from build123d import *

# Parameters (mm, degrees)
F0_R     = 17.283329
F0_R_2   = 8.664102
F1_DEPTH = 30


with BuildPart() as f1:
    # F0 (on Front) → F1 (new body)
    with BuildSketch(Plane.XZ):
        with BuildLine():
            ThreePointArc((-53.428299, -27.878553), (-36.62345, -18.213297), (-29.982977, 0))
            ThreePointArc((-29.982977, 0), (-36.62345, 18.213297), (-53.428299, 27.878553))
            ThreePointArc((-53.428299, 27.878553), (-86.578354, 0), (-53.428299, -27.878553))
        make_face()
        with Locations((-58.280665, 0)):
            Circle(F0_R, mode=Mode.SUBTRACT)
        with BuildLine():
            ThreePointArc((-53.428299, 27.878553), (-36.62345, 18.213297), (-29.982977, 0))
            ThreePointArc((-29.982977, 0), (-36.62345, -18.213297), (-53.428299, -27.878553))
            Line((-53.428299, -27.878553), (59.125109, -15.380887))
            ThreePointArc((59.125109, -15.380887), (41.996, -1.293634), (56.538776, 15.450461))
            Line((56.538776, 15.450461), (-53.428299, 27.878553))
        make_face()
        with BuildLine():
            ThreePointArc((72.892666, 0), (68.044897, 11.249072), (56.538776, 15.450461))
            ThreePointArc((56.538776, 15.450461), (41.996, -1.293634), (59.125109, -15.380887))
            ThreePointArc((59.125109, -15.380887), (68.948042, -10.321305), (72.892666, 0))
        make_face()
        with Locations((57.417251, 0)):
            Circle(F0_R_2, mode=Mode.SUBTRACT)
    extrude(amount=F1_DEPTH)


solid = f1.part
Work out the finished part from the listing and answer in its coordinate system (mm). Give positions to 0.01 mm unless a question says otherwise; leave off trailing zeros. Order: outer loops, then holes, each group sorted by start corner. A loop starts at its lowest first (then second) coordinate and runs counter-clockwise, first axis right, second up. Notation, with made-up numbers: (24, 82) -> (77, 82) arc R13 ccw to (77, 106) -> close; hole circle Ø2 at (15.5, -26). An arc over 180 degrees is marked (long way). One line per item, written item: value.
Item 1: Find section D-D, the plane x = -7.5. Give the vertices of the cut face in (y, z).
Answer sheet:
outline: (-30, -22.78) -> (0, -22.78) -> (0, 22.69) -> (-30, 22.69) -> close
Item 2: Determine the mould class of faces 1 (the flat face through (-8, -30, 0)), 2 (the cylindrical face through (55.54, -14.79, -8.46)), 3 (the flat face through (2.061, -14.79, -21.717)) for opening direction X: released by +X, released by -X, zero draft, split by the parting line, or undercut.
Answer sheet:
face 1: zero draft
face 2: undercut
face 3: released by +X
Item 3: Straight lines are drawn through the part: probe 1 along X at (y, z) = (-17, -3); probe 2 along X at (y, z) = (-27.5, -9); probe 3 along X at (y, z) = (-3.5, -6). For each, find the intervals that lie inside material, in ascending order.
Answer sheet:
probe 1: -86.42 to -75.3, -41.26 to 49.29, 65.55 to 72.6
probe 2: -85.11 to -73.04, -43.53 to 70.01
probe 3: -85.93 to -74.49, -42.07 to 51.17, 63.67 to 71.68
Item 4: Flat-ended cylindrical pins translate along their axes: P1, Ø1.5, axis at y = -4.5, z = 15, coming from the -X side; P2, Ø3, axis at x = 26, y = -6, coming from the -Z side; P3, Ø8, axis at x = -17.5, y = -13, coming from the -Z side. Find the tip coordinate at first contact, or state that the pin passes through.
Answer sheet:
P1: x = -82.73
P2: z = -19.23
P3: z = -24.33
Item 5: Find section B-B, the plane x = -48.5. Give the vertices of the cut face in (y, z), plus the area to 3 significant figures.
Answer sheet:
outline: (-30, -27.33) -> (0, -27.33) -> (0, -14.25) -> (-30, -14.25) -> close; (-30, 14.25) -> (0, 14.25) -> (0, 27.32) -> (-30, 27.32) -> close
area: 785 mm²
Item 6: Find section A-A, the plane y = -24.25. Give the vertices of the cut face in (x, z), plus the area to 3 significant figures.
Answer sheet:
outline: (-53.43, -27.88) -> (59.13, -15.38) arc R15.48 ccw to (72.89, 0) arc R15.48 ccw to (56.54, 15.45) -> (-53.43, 27.88) arc R28.3 ccw (long way) to start; hole circle Ø34.57 at (-58.28, 0); hole circle Ø17.33 at (57.42, 0)
area: 5,540 mm²
Item 7: Find section C-C, the plane z = 14. Give the vertices of the cut face in (x, y), plus the area to 3 significant figures.
Answer sheet:
outline: (-82.87, -30) -> (-68.42, -30) -> (-68.42, 0) -> (-82.87, 0) -> close; (-48.15, -30) -> (64.01, -30) -> (64.01, 0) -> (-48.15, 0) -> close
area: 3,800 mm²
